CAD build for the part. Positions are in the model's coordinates, mm. A direction names the side the tool comes from. Give positions to 0.01 mm unless a question says otherwise; leave off trailing zeros. Write each loop counter-clockwise with the first axis right and the second up, starting at its lowest first coordinate (ties: lowest second). Pieces come first, ordered by that corner, then holes. Notation, with made-up numbers: (41.25, 63.5) - (81.25, 63.5) arc R4 ccw to (81.25, 68.5) - close; hole circle Ø8 at (-38.5, 3.25). An arc over 180 degrees is marked (long way). Put each result on its own line as item: value. Start each with the question number.
1. Drop flat-ended pins along their axis: pin 1 (6 mm diameter, centred on y = -5, z = -5.5, fed in from +X); pin 2 (1.5 mm diameter, centred on x = 2, z = -22.5, fed in from -Y); pin 3 (3 mm diameter, centred on x = 1, y = 0, fed in from -Z). Give the stop position or say it passes through.
2. Mould opens along X. For faces 4 (the cylindrical face through (5.158, -3.955, -48.953)), 5 (the flat face through (-1.5, -2.6, -50.8)), 6 (the flat face through (0, 0, 0)) say: +X half, -X half, draft (parallel to the pull), parting line (faces both ways), or undercut.
3. Tool access for faces 1 (the cylindrical face through (-0.867, -3.905, -22.563)), 2 (the flat face through (-3, -3, -53)), 3 (the flat face through (-1.5, 2.6, -50.8)): list every direction of +Z, -Z, +X, -X, +Y, -Y with a clear straight run to the whole face (end or side of a thin tool).
4. Cut at C-C on z = -20.5. List the corners of the cut face in (x, y), and give its area (3 significant figures).
5. Cut at B-B on z = -47. List the corners of the cut face in (x, y).
6. Cut at A-A on y = 0. List the corners of the cut face in (x, z).
7. Wall check: line 1 (Y direction, x = 0, z = -28); line 2 (Z direction, x = 3, y = -4); line 3 (Y direction, x = -1.25, z = -49). Give the ranges that are in metal, low to high.
from build123d import *

# Parameters (mm, degrees)
SKETCH1_R            = 4
EXTRUDE1_DEPTH       = 45
SKETCH6_R            = 6.5
EXTRUDE2_DEPTH       = 8
CUT_EXTRUDE1_DEPTH   = 4.5
CHAMFER1_SIZE        = 0.65
SKETCH10_R           = 4
PARTIAL_THREAD_DEPTH = 17
CHAMFER2_SIZE        = 0.16


with BuildPart() as part:
    # Sketch1 → Extrude1 (new body)
    with BuildSketch(Plane.XY):
        Circle(SKETCH1_R)
    extrude(amount=-EXTRUDE1_DEPTH)

    # Sketch4 → Cut-Revolve1 (revolve, cut)
    with BuildSketch(Plane(origin=(0, 0, 0), x_dir=(0, 0, -1), z_dir=(1, 0, 0)), mode=Mode.PRIVATE) as cut_revolve1_sk:
        Polygon((0.746350386, 4), (0, 2.934101184), (0, 4), align=None)
    revolve(cut_revolve1_sk.sketch.rotate(Axis((0, 0, 0), (0, 0, -1)), 90), axis=Axis((0, 0, 0), (0, 0, -1)), mode=Mode.SUBTRACT)

    # Sketch6 → Extrude2 (add)
    with BuildSketch(Plane(origin=(0, 0, -45), x_dir=(-1, 0, 0), z_dir=(0, 0, -1))):
        Circle(SKETCH6_R)
    extrude(amount=EXTRUDE2_DEPTH)

    # Sketch7 → Cut-Extrude1 (cut)
    with BuildSketch(Plane(origin=(0, 0, -53), x_dir=(-1, 0, 0), z_dir=(0, 0, -1))):
        Polygon((0, 3.464101615), (-3, 1.732050808), (-3, -1.732050808), (0, -3.464101615), (3, -1.732050808), (3, 1.732050808), align=None)
    extrude(amount=-CUT_EXTRUDE1_DEPTH, mode=Mode.SUBTRACT)

    # Cut-Extrude2 cone 1 section (through the dimple's axis) → Cut-Extrude2 (revolve, cut)
    with BuildSketch(Plane(origin=(0, 0, -53), x_dir=(0, 1, 0), z_dir=(1, 0, 0))):
        Polygon((0, 0), (3.464101615, 0), (0, 3.464101615), align=None)
    revolve(axis=Axis((0, 0, -53), (0, 0, 1)), mode=Mode.SUBTRACT)

    # Chamfer1
    chamfer1_edges = [part.edges().sort_by_distance(p)[0] for p in [
        (6.5, 0, -45),
        (6.5, 0, -53),
    ]]
    chamfer(chamfer1_edges, length=CHAMFER1_SIZE)


with BuildPart() as body_2:
    # Sketch10 → partial thread (new body)
    with BuildSketch(Plane.XY.offset(-45)):
        Circle(SKETCH10_R)
    extrude(amount=PARTIAL_THREAD_DEPTH)

    # Chamfer2
    chamfer2_edges = [body_2.edges().sort_by_distance(p)[0] for p in [
        (-4, 0, -28),
    ]]
    chamfer(chamfer2_edges, length=CHAMFER2_SIZE)


with BuildPart() as part_1:
    add(part.part)

    # Combine1: union body 2
    add(body_2.part)


solid = part_1.part
Report:
1. pin 1: stops at x = 3.46
1. pin 2: stops at y = -3.8
1. pin 3: stops at z = -48.5
2. face 4: parting line
2. face 5: undercut
2. face 6: draft
3. face 1: +Z
3. face 2: -Z, +X, -X, +Y, -Y
3. face 3: -Z
4. outline: circle Ø8 at (0, 0)
4. area: 50.3 mm²
5. outline: circle Ø13 at (0, 0)
6. outline: (-6.5, -52.35) - (-5.85, -53) - (-3.46, -53) - (-3, -52.54) - (-3, -48.5) - (3, -48.5) - (3, -52.54) - (3.46, -53) - (5.85, -53) - (6.5, -52.35) - (6.5, -45.65) - (5.85, -45) - (4, -45) - (4, -0.75) - (2.93, 0) - (-2.93, 0) - (-4, -0.75) - (-4, -45) - (-5.85, -45) - (-6.5, -45.65) - close
7. line 1: y = -4 to 4
7. line 2: z = -53 to -45
7. line 3: y = -6.38 to -2.74, 2.74 to 6.38
